CAD build for the part. Positions are in the model's coordinates, mm. Face numbers are marked on the shaded views. A direction names the side the tool comes from. Give positions to 0.01 mm unless a question says otherwise; leave off trailing zeros. Order: outer loops, then holes, each group sorted by start corner. A loop starts at its lowest first (then second) coordinate and runs counter-clockwise, first axis right, second up. Notation, with made-up numbers: M 23.25,-1 L 78.25,-1 A36 ccw 78.25,38 Z; hole C -18.5,49.25 d2. An arc over 180 degrees is marked long. Put each result on its own line as item: value. Start each with the question number.
1) Cut at B-B (x = 0). Write the cut outline in (y, z).
2) Cut at D-D (z = 6). Write the cut outline in (x, y), and give its area (3 significant figures).
3) Cut at A-A (z = 0). Write the cut outline in (x, y), and give its area (3 significant figures).
4) Tool access for the marked faces 1, 2, 3 and 4: list every direction of +Z, -Z, +X, -X, +Y, -Y with a clear straight run to the whole face (end or side of a thin tool).
5) Cut at C-C (y = 11.25). Write the cut outline in (x, z), and give its area (3 significant figures).
6) Two-plate mould, pull along X, no slides. Class the marked faces 5, 6 and 7: released by +X, released by -X, zero draft, split by the parting line, or undercut.
7) Drill centre lines: line 1 (X direction, y = 1.8, z = 0); line 2 (Z direction, x = 0, y = 2); line 3 (Y direction, x = -4.75, z = -5). Where is each one in solid material? Low to high. Write a range as [from, to].
8) Pin check, flat tips, straight feed: pin 1 (4 mm diameter, centred on y = 11, z = 6.5, fed in from +X); pin 2 (5 mm diameter, centred on y = 2.5, z = -3, fed in from +X); pin 3 (5 mm diameter, centred on y = 3, z = 6, fed in from -X). Stop position of each tip, or through.
Autodesk Fusion 360 part; units mm, degrees
sketch "Sketch1" plane through (0, 0, 0) normal (0, 1, 0) x (1, 0, 0)
  arc A0 (-1.5, 2) -> (1.5, 2) centre (0, 0) ccw
  line L0 (1.5, 2) -> (-1.5, 2)
  circle A1 centre (0, 0) radius 9.5
  dimension "d1" = 3
  dimension "d2" = 2.5
  dimension "d3" = 19
extrude "Extrude1" add sketch "Sketch1" along normal blind 4
sketch "Sketch2" plane through (0, 4, 0) normal (0, 1, 0) x (-1, 0, 0)
  arc A0 (1.5, -2) -> (-1.5, -2) centre (0, 0) ccw
  line L0 (1.5, -2) -> (-1.5, -2)
  line L1 (4.5, -7) -> (-4.5, -7) construction
  line L2 (0, -14.5329) -> (0, 17.7812) construction
  circle A1 centre (0, 0) radius 9.5 construction
  circle A2 centre (0, 0) radius 7 construction
  line L3 (6.7857, -6.6486) -> (5, -4.899)
  line L4 (-5, -4.899) -> (-6.7857, -6.6486)
  arc A3 (-5, -4.899) -> (5, -4.899) centre (0, 0) ccw
  arc A4 (-6.7857, -6.6486) -> (6.7857, -6.6486) centre (0, 0) ccw
  dimension "d6" = 3
  dimension "d7" = 2.5
  dimension "d8" = 9
  dimension "d9" = 4.5
  dimension "d10" = 14
  dimension "d14" = 10
  dimension "d15" = 7
  dimension "d16" = 9.5
extrude "Extrude2" add sketch "Sketch2" along normal blind 8.5 contours L3 L4 A3 A4
mirror "Mirror1" about plane through (0, 0, 0) normal (0, 0, 1) of "Extrude2"
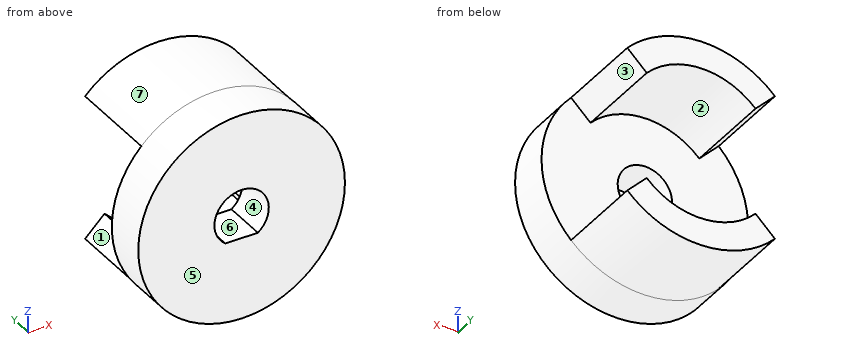
Solution:
1. outline: M 0,-9.5 L 12.5,-9.5 L 12.5,-7 L 4,-7 L 4,-2 L 0,-2 Z; M 0,2.5 L 4,2.5 L 4,7 L 12.5,7 L 12.5,9.5 L 0,9.5 Z
2. outline: M -7.37,0 L 7.37,0 L 7.37,4 L 6.12,4 L 6.12,12.5 L 3.61,12.5 L 3.61,4 L -3.61,4 L -3.61,12.5 L -6.12,12.5 L -6.12,4 L -7.37,4 Z
2. area: 102 mm²
3. outline: M -9.5,0 L -2.5,0 L -2.5,4 L -9.5,4 Z; M 2.5,0 L 9.5,0 L 9.5,4 L 2.5,4 Z
3. area: 56.0 mm²
4. face 1: -X, +Y
4. face 2: +Y
4. face 3: +X, +Y
4. face 4: +Y, -Y
5. outline: M -6.79,-6.65 A9.5 ccw 6.79,-6.65 L 5,-4.9 A7 cw -5,-4.9 Z; M -6.79,6.65 L -5,4.9 A7 cw 5,4.9 L 6.79,6.65 A9.5 ccw Z
5. area: 65.6 mm²
6. face 5: zero draft
6. face 6: undercut
6. face 7: split by the parting line
7. line 1: [-9.5, -2.5], [2.5, 9.5]
7. line 2: [-9.5, -2], [2.5, 9.5]
7. line 3: [0, 4]
8. pin 1: x = 6.79
8. pin 2: x = 9.49
8. pin 3: x = -8.83
